```python
from build123d import *

# Parameters (mm, degrees)
F0_R          = 52.5
F0_R_2        = 50.5
F0_R_3        = 47.5
F1_DEPTH      = 10
F1_DEPTH_BACK = 4
F0_R_4        = 53.5
F2_DEPTH      = 70
F2_DEPTH_BACK = 4
F4_R          = 52.5
F4_R_2        = 48
F5_DEPTH      = 10
F8_R          = 5


# Not quite as in the source:
# - the program builds the solid bodies; features that only make, move or delete a surface that nothing else refers to are left out


with BuildPart() as f1:
    # F0 (on Top) → F1 (new body, two sides)
    with BuildSketch(Plane.XY) as f1_sk:
        Circle(F0_R)
        Circle(F0_R_2, mode=Mode.SUBTRACT)
        Circle(F0_R_2)
        Circle(F0_R_3, mode=Mode.SUBTRACT)
    extrude(amount=F1_DEPTH)
    extrude(f1_sk.sketch, amount=-F1_DEPTH_BACK)

    # F0 (on Top) → F2 (join, two sides)
    with BuildSketch(Plane.XY) as f2_sk:
        Circle(F0_R_4)
        Circle(F0_R, mode=Mode.SUBTRACT)
    extrude(amount=F2_DEPTH)
    extrude(f2_sk.sketch, amount=-F2_DEPTH_BACK)

    # F4 (on offset) → F5 (join)
    with BuildSketch(Plane.XY.offset(60)):
        Circle(F4_R)
        Circle(F4_R_2, mode=Mode.SUBTRACT)
    extrude(amount=F5_DEPTH)

    # F8
    f8_edges = [f1.edges().sort_by_distance(p)[0] for p in [
        (-53.5, 0, -4),
    ]]
    fillet(f8_edges, radius=F8_R)


solid = f1.part
```
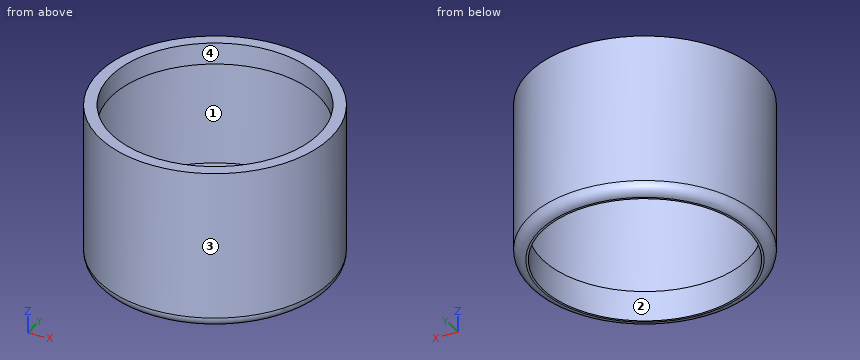
Work out the finished part from the listing and answer in its coordinate system (mm). Face numbers are marked on the shaded views. A direction names the side the tool comes from. Round coordinates to 2 decimals unless told otherwise and drop trailing zeros. Loops run counter-clockwise (first coordinate to the right, second up) from the corner with the lowest first, then second, coordinate; pieces in that order, holes last.
(1) The mould has two halves that part along Y. Classify the marked faces 3 and 4: pulls with the +Y half, pulls with the -Y half, needs draft (parallel to the pull), parting line crosses it, or undercut.
Computed values:
face 3: parting line crosses it
face 4: undercut
(2) The part is cut by section C-C, the plane z = 17. Give the vertices of the cut face in (x, y).
Computed values:
outline: circle Ø107 at (0, 0); hole circle Ø105 at (0, 0)
(3) Each of these flat-tipped pins is pushed along its axis until it touches: P1, Ø1, axis at y = 42.5, z = 50, coming from the -X side; P2, Ø2, axis at y = 37.5, z = 52.5, coming from the -X side; P3, Ø8, axis at x = 31, z = 52, coming from the -Y side; P4, Ø12, axis at x = 27, y = -41, coming from the -Z side. Where does it stop, or does it pass through?
Computed values:
P1: stops at x = -33.14
P2: stops at x = -39.12
P3: stops at y = -46.19
P4: stops at z = -4
(4) For the marked faces 1 and 2, determine the directions among +Z, -Z, +X, -X, +Y, -Y from which every point of the face is accessible in a straight line to the end or side of a thin tool.
Computed values:
face 1: none
face 2: +Z, -Z
(5) The part is cut by section A-A, the plane x = 0. Give the vertices of the cut face in (y, z), and give its area (3 significant figures).
Computed values:
outline: (-53.5, 1) arc R5 ccw to (-48.5, -4) - (-47.5, -4) - (-47.5, 10) - (-52.5, 10) - (-52.5, 60) - (-48, 60) - (-48, 70) - (-53.5, 70) - close; (47.5, -4) - (48.5, -4) arc R5 ccw to (53.5, 1) - (53.5, 70) - (48, 70) - (48, 60) - (52.5, 60) - (52.5, 10) - (47.5, 10) - close
area: 367 mm2
(6) Find the intervals of material crossed by L1, parallel to X at y = -1.5, z = 57; L2, parallel to Y at x = 0, z = 22.5; L3, parallel to X at y = 24, z = 38, in increasing order.
Computed values:
L1: x = -53.48 to -52.48, 52.48 to 53.48
L2: y = -53.5 to -52.5, 52.5 to 53.5
L3: x = -47.81 to -46.69, 46.69 to 47.81
